Here's how the part is built. I have some questions about the finished solid (model axes, mm). A direction names the side the tool comes from. Round coordinates to 2 decimals unless told otherwise and drop trailing zeros. Loops run counter-clockwise (first coordinate to the right, second up) from the corner with the lowest first, then second, coordinate; pieces in that order, holes last. Notation, with made-up numbers: (40.5, 82) - (98.5, 82) arc R35 ccw to (98.5, 116) - close; hole circle Ø10 at (-5, 27). An arc over 180 degrees is marked (long way). Return JSON: item names as keys, results as strings. Group by question number.
```python
from build123d import *

# Parameters (mm, degrees)
F0_W   = 25.4
F0_H   = 25.4
F0_W_2 = 19.05
F0_H_2 = 19.05


with BuildPart() as f2:
    # F2: sweep along a path in F1
    with BuildLine(Plane.YZ) as f2_path:
        Line((0, 0), (0, 152.4))
        Line((0, 152.4), (76.2, 20.4177284633))
        Line((76.2, 20.4177284633), (76.2, 172.8177284633))
        Line((76.2, 172.8177284633), (0, 304.8))
    # F0 (on Top) → F2 (sweep)
    with BuildSketch(Plane.XY):
        Rectangle(F0_W, F0_H)
        Rectangle(F0_W_2, F0_H_2, mode=Mode.SUBTRACT)
    sweep(path=f2_path.line, transition=Transition.RIGHT)


solid = f2.part
```
Q1. Imagine slicing it at C-C, the plane z = 142. List the corners of the cut face in (x, y) for me (3 decimals).
Q2. Imagine slicing it at B-B, the plane y = 27.5. List the corners of the cut face in (x, z) for me (3 decimals).
Q3. If we mould it in two halves opening along Z, with no side actions, what happens to faces 1 (the flat face through (0, 63.5, 119)), 2 (the flat face through (0.18, 51.33, 38.09)), 3 (the flat face through (0, 9.525, 59)), 4 (the flat face through (-0.178, 25.933, 132.882))? For each: +Z half, -Z half, draft (parallel to the pull), parting line (faces both ways), or undercut.
Q4. Imagine slicing it at D-D, the plane z = 93.5. List the corners of the cut face in (x, y) for me (3 decimals), and give its area (3 significant figures).
Q5. Please list where these lines run through material, in increasing order: line 1 (X direction, y = 79.5, z = 158) (3 decimals); line 2 (Z direction, x = 3.75, y = 22); line 3 (Y direction, x = 5.75, z = 62.5) (3 decimals).
Q6. For faces 5 (the flat face through (9.525, 28, 113)), 6 (the flat face through (0, -9.525, 95)), 7 (the flat face through (0, 12.7, 53)), which set-ups out of +Z, -Z, +X, -X, +Y, -Y let a thin tool reach every point of the face, with its end or its side?
Q7. Will these pins go through, and if not, where does the flat tip stop? pin 1 Ø12 at (y, z) = (45.5, 261) entering from +X; pin 2 Ø6 at (x, y) = (7, 19.5) entering from +Z; pin 3 Ø2 at (x, y) = (7, 54) entering from -Z; pin 4 Ø12.5 at (x, y) = (-6, -5.5) entering from -Z.
Output values:
{
 "1": {"outline": "(-12.7, -12.7) - (12.7, -12.7) - (12.7, 20.669) - (-12.7, 20.669) - close; (-12.7, 63.5) - (12.7, 63.5) - (12.7, 88.9) - (-12.7, 88.9) - close; hole (-9.525, -9.525) - (9.525, -9.525) - (9.525, 17.003) - (-9.525, 17.003) - close; hole (-9.525, 66.675) - (9.525, 66.675) - (9.525, 85.725) - (-9.525, 85.725) - close"},
 "2": {"outline": "(-12.7, 79.369) - (12.7, 79.369) - (12.7, 130.169) - (-12.7, 130.169) - close; (-12.7, 231.769) - (12.7, 231.769) - (12.7, 282.569) - (-12.7, 282.569) - close; hole (-9.525, 85.719) - (9.525, 85.719) - (9.525, 123.819) - (-9.525, 123.819) - close; hole (-9.525, 238.119) - (9.525, 238.119) - (9.525, 276.219) - (-9.525, 276.219) - close"},
 "3": {"face 1": "undercut", "face 2": "-Z half", "face 3": "draft", "face 4": "undercut"},
 "4": {"outline": "(-12.7, -12.7) - (12.7, -12.7) - (12.7, 12.7) - (-12.7, 12.7) - close; (-12.7, 19.341) - (12.7, 19.341) - (12.7, 48.671) - (-12.7, 48.671) - close; (-12.7, 63.5) - (12.7, 63.5) - (12.7, 88.9) - (-12.7, 88.9) - close; hole (-9.525, -9.525) - (9.525, -9.525) - (9.525, 9.525) - (-9.525, 9.525) - close; hole (-9.525, 23.007) - (9.525, 23.007) - (9.525, 45.004) - (-9.525, 45.004) - close; hole (-9.525, 66.675) - (9.525, 66.675) - (9.525, 85.725) - (-9.525, 85.725) - close", "area": "890 mm^2"},
 "5": {"line 1": "x = -12.7 to -9.525, 9.525 to 12.7", "line 2": "z = 88.89 to 95.24, 133.34 to 139.69, 241.29 to 247.64, 285.74 to 292.09", "line 3": "y = -12.7 to -9.525, 9.525 to 12.7, 37.239 to 40.905, 62.902 to 66.675, 85.725 to 88.9"},
 "6": {"face 5": "none", "face 6": "-Z", "face 7": "-Z, +X, -X"},
 "7": {"pin 1": "stops at x = 12.7", "pin 2": "stops at z = 301.62", "pin 3": "stops at z = 31.74", "pin 4": "stops at z = 0"}
}
